Autodesk Fusion 360 part; units mm, degrees
sketch "Sketch1" plane through (0, 0, 0) normal (0, 0, 1) x (1, 0, 0)
  line L0 (0, 0) -> (0, 50)
  line L1 (0, 50) -> (10, 50)
  line L2 (30, 50) -> (30, 75)
  line L3 (30, 75) -> (30, 35)
  arc A0 (30, 75) -> (10, 50) centre (35.3698, 50.2041) ccw
  line L4 (30, 35) -> (125, 35)
  line L5 (125, 35) -> (125, 50)
  line L6 (125, 50) -> (150, 50)
  line L7 (150, 50) -> (150, 0)
  line L8 (150, 0) -> (0, 0)
extrude "Extrude1" add sketch "Sketch1" along normal blind 50
sketch "Sketch2" plane through (150, 0, 0) normal (1, 0, 0) x (0, 1, 0)
  line L0 (0, 0) -> (50, 0)
  line L1 (50, 0) -> (50, 50)
  line L2 (50, 50) -> (0, 50)
  line L3 (0, 50) -> (0, 0)
  circle A0 centre (50, 25) radius 15
extrude "Extrude2" add sketch "Sketch2" against normal blind 25 contours L1 A0 picked at (54.9491, 25.7116)
sketch "Sketch3" plane through (0, 35, 0) normal (0, 1, 0) x (-1, 0, 0)
  line L0 (-125, 0) -> (-30, 0)
  line L1 (-30, 0) -> (-30, 50)
  line L2 (-30, 50) -> (-125, 50)
  line L3 (-125, 50) -> (-125, 0)
  line L4 (-125, 15) -> (-30, 15)
  line L5 (-30, 15) -> (-30, 35)
  line L6 (-30, 35) -> (-125, 35)
  line L7 (-125, 35) -> (-125, 15)
extrude "Extrude3" add sketch "Sketch3" along normal blind 10 contours L1 L3 L4 L5 L6 L7
sketch "Sketch4" plane through (0, 0, 0) normal (0, -1, 0) x (1, 0, 0)
  line L0 (0, 0) -> (150, 0)
  line L1 (150, 0) -> (150, 50)
  line L2 (150, 50) -> (0, 50)
  line L3 (0, 50) -> (0, 0)
  line L4 (0, 10) -> (150, 10)
  line L5 (150, 10) -> (150, 40)
  line L6 (150, 40) -> (0, 40)
  line L7 (0, 40) -> (0, 10)
  line L8 (150, 35) -> (0, 35)
  line L9 (0, 35) -> (0, 15)
  line L10 (0, 15) -> (150, 15)
  line L11 (150, 15) -> (150, 35)
extrude "Extrude4" cut sketch "Sketch4" against normal blind 35 contours L1 L3 L5 L7 L8 L9 L10 L11
extrude "Extrude5" cut sketch "Sketch4" against normal blind 20 contours L1 L3 L4 L5 L7 L10 | L1 L3 L5 L6 L7 L8
Geometry check sheet. Reference: the model listing, model coordinates, mm. A direction names the side the tool comes from. Round coordinates to 2 decimals unless told otherwise and drop trailing zeros. Order: outer loops, then holes, each group sorted by start corner. A loop starts at its lowest first (then second) coordinate and runs counter-clockwise, first axis right, second up. Notation, with made-up numbers: (2.5, 42) - (60.5, 42) arc R8 cw to (60.5, 57) - close; hole circle Ø7 at (89.25, 18.5). An arc over 180 degrees is marked (long way). Use a Markdown table: item, result. Add a question column.
(1) Tool access check on faces 4 (the flat face through (5, 50, 25)), 5 (the flat face through (74, 20, 13)), 6 (the flat face through (137, 50, 45)). Record the directions out of +Z, -Z, +X, -X, +Y, -Y that give a thin tool (end or side, any length) a straight path to the whole face; none if there is none.
(2) Depth check by flat-ended pin: pin 1 (1.5 mm diameter, centred on x = 31, y = 46.5, fed in from +Z); pin 2 (1.5 mm diameter, centred on y = 67, z = 16.5, fed in from +X); pin 3 (6 mm diameter, centred on x = 59, z = 24.5, fed in from +Y); pin 4 (8 mm diameter, centred on x = 143.5, z = 46, fed in from +Y). Enter the tip coordinate at first touch or a pass-through.
(3) Sectioned sample at D-D, the plane z = 41.5. Enter the section's corners in (x, y).
(4) Release check for a two-part mould opening along Z. For faces 1 (the flat face through (76, 0, 45)), 2 (the flat face through (74, 35, 25)), 3 (the flat face through (77, 40, 35)) record: pulls with the +Z half, pulls with the -Z half, needs draft (parallel to the pull), parting line crosses it, or undercut.
(5) Sectioned sample at C-C, the plane y = 28.5. Enter the section's corners in (x, z).
(6) Sectioned sample at B-B, the plane z = 25. Enter the section's corners in (x, y).
(7) Material ranges on line 1 along X through (y, z) = (41.5, 47); line 2 along Z through (x, y) = (75, 14); line 3 along Z through (x, y) = (65, 23.5), recorded low to high. Write a range as [from, to].
Answers below:
| question | item | result |
|---|---|---|
| 1 | face 4 | +Z, -Z, -X, +Y |
| 1 | face 5 | +X, -X, -Y |
| 1 | face 6 | +Z, +X, +Y |
| 2 | pin 1 | through |
| 2 | pin 2 | x = 30 |
| 2 | pin 3 | y = 45 |
| 2 | pin 4 | y = 50 |
| 3 | outline | (0, 0) - (150, 0) - (150, 50) - (125, 50) - (125, 35) - (30, 35) - (30, 75) arc R25.37 ccw to (10, 50) - (0, 50) - close |
| 4 | face 1 | needs draft |
| 4 | face 2 | undercut |
| 4 | face 3 | pulls with the +Z half |
| 5 | outline | (0, 0) - (150, 0) - (150, 15) - (0, 15) - close; (0, 35) - (150, 35) - (150, 50) - (0, 50) - close |
| 6 | outline | (0, 35) - (150, 35) - (150, 65) - (125, 65) - (125, 45) - (30, 45) - (30, 75) arc R25.37 ccw to (10, 50) - (0, 50) - close |
| 7 | line 1 | [0, 30], [125, 150] |
| 7 | line 2 | [0, 10], [40, 50] |
| 7 | line 3 | [0, 15], [35, 50] |
